Geometry: final body of the model. Coordinates: model frame, mm. Face numbers are marked on the shaded views. A direction names the side the tool comes from. Give positions to 0.01 mm unless a question says otherwise; leave off trailing zeros. Write each loop counter-clockwise with the first axis right and the second up, starting at its lowest first coordinate (ties: lowest second). Pieces come first, ordered by that corner, then holes. Notation, with made-up numbers: (88, -27) -> (122, -27) arc R22 cw to (122, 6) -> close; hole circle Ø6 at (14, 47). An arc over 180 degrees is marked (long way). Answer as a JSON object with one key per item and string values. Group by question number.
(1) Material intervals for probe 1 along Y at (x, z) = (23.5, -26); probe 2 along X at (y, z) = (122, -110); probe 3 along X at (y, z) = (115, -135.75), sorted ascending.
(2) Section query C-C on z = -134. Output: boundary loops of the cut face in (x, y).
(3) Set-up query: the marked faces 4, 5, 6, 7 and 8. Return all of +Z, -Z, +X, -X, +Y, -Y with unobstructed straight access to the full face (end or side cutting, diameter ignored); none if empty.
(4) Section query A-A on x = 87.5. Output: boundary loops of the cut face in (y, z), plus the area to 3 significant figures.
(5) Section query B-B on x = 38.5. Output: boundary loops of the cut face in (y, z).
(6) Contact query for flat-ended pins moving along their axis: pin 1 Ø6.5 at (x, z) = (110, -110) entering from +Y; pin 2 Ø17.5 at (y, z) = (103.5, -131.5) entering from +X; pin 3 Ø1.5 at (x, y) = (73, 56.5) entering from -Z. Output: stop coordinate, or through.
(7) Draft query along Y for the marked faces 1, 2 and 3. Return one class per face: +Y half, -Y half, draft (parallel to the pull), parting line (faces both ways), or undercut.
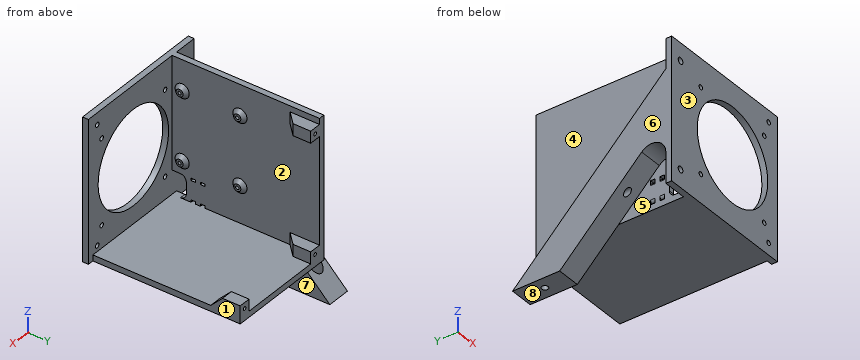
from build123d import *

# Parameters (mm, degrees)
SKETCH1_W               = 120
SKETCH1_H               = 120
BOSS_EXTRUDE1_DEPTH     = 5
SKETCH5_W               = 5
SKETCH5_H               = 120
BOSS_EXTRUDE3_DEPTH     = 125
SKETCH15_W              = 90
SKETCH15_H              = 5
BOSS_EXTRUDE9_DEPTH     = 125
SKETCH3_R               = 40
CUT_EXTRUDE1_DEPTH      = 15
SKETCH4_R               = 1.95
CUT_EXTRUDE2_DEPTH      = 15
SKETCH6_R               = 3
BOSS_EXTRUDE4_DEPTH     = 3
SKETCH7_R               = 1.45
CUT_EXTRUDE3_DEPTH      = 7
BOSS_EXTRUDE8_DEPTH     = 20
CUT_EXTRUDE6_DEPTH      = 236.212669727
CUT_EXTRUDE6_DEPTH_BACK = 236.212669727
SKETCH12_R              = 2.65
CHAMFER3_SIZE           = 3
SKETCH17_W              = 10
SKETCH17_H              = 10
BOSS_EXTRUDE10_DEPTH    = 15
CHAMFER4_SIZE           = 10
SKETCH18_R              = 2
CUT_EXTRUDE8_DEPTH      = 15
SKETCH19_R              = 1.45
CUT_EXTRUDE9_DEPTH      = 15
FILLET4_R               = 12
SKETCH20_R              = 2.65
CUT_EXTRUDE10_DEPTH     = 239.012604708
SKETCH21_R              = 5.5
CUT_EXTRUDE11_DEPTH     = 235.787137637
FILLET5_R               = 5
SKETCH23_W              = 20
SKETCH23_H              = 12
SKETCH23_W_2            = 2
SKETCH23_H_2            = 4
CUT_EXTRUDE12_DEPTH     = 10
FILLET6_R               = 5
FILLET7_R               = 2


with BuildPart() as part:
    # Sketch1 → Boss-Extrude1 (new body)
    with BuildSketch(Plane(origin=(0, 0, 0), x_dir=(1, 0, 0), z_dir=(0, 1, 0))):
        with Locations((60, 60)):
            Rectangle(SKETCH1_W, SKETCH1_H)
    extrude(amount=BOSS_EXTRUDE1_DEPTH)

    # Sketch5 → Boss-Extrude3 (add)
    with BuildSketch(Plane(origin=(0, 5, 0), x_dir=(1, 0, 0), z_dir=(0, 1, 0))):
        with Locations((22.5, 60)):
            Rectangle(SKETCH5_W, SKETCH5_H)
    extrude(amount=BOSS_EXTRUDE3_DEPTH)

    # Sketch15 → Boss-Extrude9 (add)
    with BuildSketch(Plane(origin=(0, 5, 0), x_dir=(1, 0, 0), z_dir=(0, 1, 0))):
        with Locations((70, 117.5)):
            Rectangle(SKETCH15_W, SKETCH15_H)
    extrude(amount=BOSS_EXTRUDE9_DEPTH)

    # Sketch3 → Cut-Extrude1 (cut)
    with BuildSketch(Plane.XZ):
        with Locations(Location((69, -60, 0), (0, 0, 270))):
            Circle(SKETCH3_R)
    extrude(amount=-CUT_EXTRUDE1_DEPTH, mode=Mode.SUBTRACT)

    # Sketch4 → Cut-Extrude2 (cut)
    with BuildSketch(Plane.XZ):
        with Locations(Location((33, -24, 0), (0, 0, 270))):
            Circle(SKETCH4_R)
        with Locations(Location((105, -24, 0), (0, 0, 270))):
            Circle(SKETCH4_R)
        with Locations(Location((105, -96, 0), (0, 0, 270))):
            Circle(SKETCH4_R)
        with Locations(Location((33, -96, 0), (0, 0, 270))):
            Circle(SKETCH4_R)
    extrude(amount=-CUT_EXTRUDE2_DEPTH, mode=Mode.SUBTRACT)

    # Sketch6 → Boss-Extrude4 (add)
    with BuildSketch(Plane(origin=(25, 0, 0), x_dir=(0, 0, -1), z_dir=(1, 0, 0))):
        with Locations(Location((26, 62.5, 0), (0, 0, 180))):
            Circle(SKETCH6_R)
        with Locations(Location((84, 62.5, 0), (0, 0, 180))):
            Circle(SKETCH6_R)
        with Locations(Location((84, 13.5, 0), (0, 0, 180))):
            Circle(SKETCH6_R)
        with Locations(Location((26, 13.5, 0), (0, 0, 180))):
            Circle(SKETCH6_R)
    extrude(amount=BOSS_EXTRUDE4_DEPTH)

    # Sketch7 → Cut-Extrude3 (cut)
    with BuildSketch(Plane(origin=(28, 0, 0), x_dir=(0, 0, -1), z_dir=(1, 0, 0))):
        with Locations((26, 62.5)):
            Circle(SKETCH7_R)
        with Locations((84, 62.5)):
            Circle(SKETCH7_R)
        with Locations((84, 13.5)):
            Circle(SKETCH7_R)
        with Locations((26, 13.5)):
            Circle(SKETCH7_R)
    extrude(amount=-CUT_EXTRUDE3_DEPTH, mode=Mode.SUBTRACT)

    # Sketch14 → Boss-Extrude8 (add)
    with BuildSketch(Plane.ZY):
        Polygon((-25, 5), (-65, 5), (-155, 95), (-155, 135), align=None)
    extrude(amount=-BOSS_EXTRUDE8_DEPTH)

    # Sketch12 → Cut-Extrude6 (cut, two sides: drawn at the far end of the back side and taken through both)
    with BuildSketch(Plane(origin=(0, 5, 0), x_dir=(1, 0, 0), z_dir=(0, 1, 0)).offset(-CUT_EXTRUDE6_DEPTH_BACK)):
        with Locations(Location((10, 105, 0), (0, 0, 90))):
            Circle(SKETCH12_R)
        with Locations(Location((10, 15, 0), (0, 0, 270))):
            Circle(SKETCH12_R)
    extrude(amount=CUT_EXTRUDE6_DEPTH + CUT_EXTRUDE6_DEPTH_BACK, mode=Mode.SUBTRACT)

    # Chamfer3
    chamfer3_edges = [part.edges().sort_by_distance(p)[0] for p in [
        (25, 62.5, -29),
        (25, 62.5, -87),
        (25, 13.5, -87),
        (25, 13.5, -29),
    ]]
    chamfer(chamfer3_edges, length=CHAMFER3_SIZE - 0.0001)  # a hair under: the kernel refuses the full size

    # Sketch17 → Boss-Extrude10 (add)
    with BuildSketch(Plane(origin=(0, 130, 0), x_dir=(1, 0, 0), z_dir=(0, 1, 0))):
        with Locations((30, 110)):
            Rectangle(SKETCH17_W, SKETCH17_H)
        with Locations((110, 110)):
            Rectangle(SKETCH17_W, SKETCH17_H)
        with Locations((30, 10)):
            Rectangle(SKETCH17_W, SKETCH17_H)
    extrude(amount=-BOSS_EXTRUDE10_DEPTH)

    # Chamfer4
    chamfer4_edges = [part.edges().sort_by_distance(p)[0] for p in [
        (110, 115, -115),
        (25, 115, -10),
        (25, 115, -110),
    ]]
    chamfer(chamfer4_edges, length=CHAMFER4_SIZE - 0.0001)  # a hair under: the kernel refuses the full size

    # Sketch18 → Cut-Extrude8 (cut)
    with BuildSketch(Plane(origin=(0, 5, 0), x_dir=(1, 0, 0), z_dir=(0, 1, 0))):
        with Locations(Location((110, 10, 0), (0, 0, 270))):
            Circle(SKETCH18_R)
        with Locations(Location((110, 110, 0), (0, 0, 270))):
            Circle(SKETCH18_R)
    extrude(amount=-CUT_EXTRUDE8_DEPTH, mode=Mode.SUBTRACT)

    # Sketch19 → Cut-Extrude9 (cut)
    with BuildSketch(Plane(origin=(0, 130, 0), x_dir=(1, 0, 0), z_dir=(0, 1, 0))):
        with Locations(Location((30, 110, 0), (0, 0, 270))):
            Circle(SKETCH19_R)
        with Locations(Location((110, 110, 0), (0, 0, 270))):
            Circle(SKETCH19_R)
        with Locations(Location((30, 10, 0), (0, 0, 270))):
            Circle(SKETCH19_R)
    extrude(amount=-CUT_EXTRUDE9_DEPTH, mode=Mode.SUBTRACT)

    # Fillet4
    fillet4_edges = [part.edges().sort_by_distance(p)[0] for p in [
        (10, 5, -65),
    ]]
    fillet(fillet4_edges, radius=FILLET4_R)

    # Sketch20 → Cut-Extrude10 (cut, through all)
    with BuildSketch(Plane(origin=(0, 0, -155), x_dir=(-1, 0, 0), z_dir=(0, 0, -1))):
        with Locations(Location((-10, 115, 0), (0, 0, 90))):
            Circle(SKETCH20_R)
    extrude(amount=-CUT_EXTRUDE10_DEPTH, mode=Mode.SUBTRACT)

    # Sketch21 → Cut-Extrude11 (cut, through all)
    with BuildSketch(Plane(origin=(0, 0, -150), x_dir=(-1, 0, 0), z_dir=(0, 0, -1))):
        with Locations(Location((-10, 115, 0), (0, 0, 90))):
            Circle(SKETCH21_R)
    extrude(amount=-CUT_EXTRUDE11_DEPTH, mode=Mode.SUBTRACT)

    # Fillet5
    fillet5_edges = [part.edges().sort_by_distance(p)[0] for p in [
        (20, 52.5, -72.5),
    ]]
    fillet(fillet5_edges, radius=FILLET5_R)

    # Sketch23 → Cut-Extrude12 (cut)
    with BuildSketch(Plane(origin=(25, 0, 0), x_dir=(0, 0, -1), z_dir=(1, 0, 0))):
        with Locations((105, 11)):
            Rectangle(SKETCH23_W, SKETCH23_H)
        with Locations((96, 23)):
            Rectangle(SKETCH23_W_2, SKETCH23_H_2)
        with Locations((114, 23)):
            Rectangle(SKETCH23_W_2, SKETCH23_H_2)
        with Locations((114, 31)):
            Rectangle(SKETCH23_W_2, SKETCH23_H_2)
        with Locations((96, 31)):
            Rectangle(SKETCH23_W_2, SKETCH23_H_2)
    extrude(amount=-CUT_EXTRUDE12_DEPTH, mode=Mode.SUBTRACT)

    # Fillet6
    fillet6_edges = [part.edges().sort_by_distance(p)[0] for p in [
        (22.5, 17, -115),
        (22.5, 17, -95),
    ]]
    fillet(fillet6_edges, radius=FILLET6_R)

    # Fillet7
    fillet7_edges = [part.edges().sort_by_distance(p)[0] for p in [
        (20, 31, -113),
        (20, 31, -97),
        (20, 23, -113),
        (20, 23, -97),
    ]]
    fillet(fillet7_edges, radius=FILLET7_R)


solid = part.part
Answer list:
{
 "1": {"probe 1": "0 to 12.05, 14.95 to 61.05, 63.95 to 130", "probe 2": "20 to 28.55, 31.45 to 35, 105 to 108.55, 111.45 to 115", "probe 3": "0 to 4.5, 15.5 to 20"},
 "2": {"outline": "(0, 74) -> (20, 74) -> (20, 114) -> (15.41, 114) arc R5.5 cw to (4.59, 114) -> (0, 114) -> close"},
 "3": {"face 4": "+Z, -X, +Y", "face 5": "-Z, -X", "face 6": "+Z, -Z, -X, +Y, -Y", "face 7": "-Z, +X, +Y, -Y", "face 8": "-Z, +X, -X, +Y, -Y"},
 "4": {"outline": "(0, -120) -> (130, -120) -> (130, -115) -> (5, -115) -> (5, -95.46) -> (0, -95.46) -> close; (0, -24.54) -> (5, -24.54) -> (5, 0) -> (0, 0) -> close", "area": "870 mm2"},
 "5": {"outline": "(0, -120) -> (130, -120) -> (130, -115) -> (5, -115) -> (5, -85.88) -> (0, -85.88) -> close; (0, -34.12) -> (5, -34.12) -> (5, 0) -> (0, 0) -> close"},
 "6": {"pin 1": "y = 130", "pin 2": "x = 20", "pin 3": "z = -120"},
 "7": {"face 1": "draft", "face 2": "undercut", "face 3": "-Y half"}
}
